Source: CAD feature listing. Evaluate the final solid. Frame: model axes, mm. Face numbers are marked on the shaded views. A direction names the side the tool comes from. Round coordinates to 2 decimals unless told otherwise and drop trailing zeros. Order: outer loops, then holes, each group sorted by start corner. A loop starts at its lowest first (then second) coordinate and runs counter-clockwise, first axis right, second up. Notation, with made-up numbers: (60, -10) -> (89, -10) arc R18 cw to (89, 11) -> close; hole circle Ø5 at (79, 78.25). An arc over 180 degrees is marked (long way). One line per item, written item: value. Start each with the question number.
1) Section C-C (y = 7.5). Return the cut outline in (x, z), and give its area (3 significant figures).
2) Ray query, L1, parallel to Y at x = 2, z = 6.5; L2, parallel to Y at x = -1.75, z = 4.25; L3, parallel to Z at x = -5, y = -6. Return the intervals inside material, ascending.
3) Section B-B (z = 5.25). Return the cut outline in (x, y).
4) Reachability of the marked faces 1, 2, 3, 4 and 5 from +Z, -Z, +X, -X, +Y, -Y: full face, straight path, thin tool, end or side. Return the list, or none.
5) Section A-A (x = 4). Return the cut outline in (y, z).
6) Pin query (flat end, axial travel): P1, Ø2.5, axis at y = -9.5, z = 4.5, coming from the +X side; P2, Ø8, axis at x = -1.5, z = 13.5, coming from the -Y side; P3, Ø5.5, axis at x = -3, z = 5, coming from the +Y side; P4, Ø1.1, axis at y = 9.5, z = 6.5, coming from the -X side. Return the tip coordinate at first contact, or that it passes through.
7) Section D-D (x = 1.5). Return the cut outline in (y, z).
8) Mould query, pull axis Y, two halves, no side actions, for the marked faces 6, 7, 8 and 9. Classes: pulls with the +Y half, pulls with the -Y half, needs draft (parallel to the pull), parting line crosses it, or undercut.
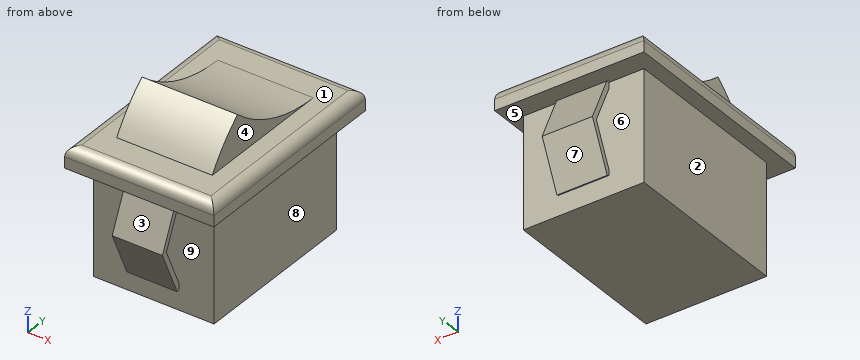
```python
from build123d import *

# Parameters (mm, degrees)
ESQUISSE1_W        = 12
ESQUISSE1_H        = 17
BOSS_EXTRU_1_DEPTH = 11
ESQUISSE2_W        = 14.823529412
ESQUISSE2_H        = 21
BOSS_EXTRU_2_DEPTH = 2.1
BOSS_EXTRU_3_DEPTH = 4.75
EXTRU_MINCE1_DEPTH = 2.5
CONG_1_R           = 1


with BuildPart() as part:
    # Esquisse1 → Boss.-Extru.1 (new body)
    with BuildSketch(Plane.XY):
        Rectangle(ESQUISSE1_W, ESQUISSE1_H)
    extrude(amount=BOSS_EXTRU_1_DEPTH)

    # Esquisse2 → Boss.-Extru.2 (add)
    with BuildSketch(Plane.XY.offset(11)):
        Rectangle(ESQUISSE2_W, ESQUISSE2_H)
    extrude(amount=BOSS_EXTRU_2_DEPTH)

    # Esquisse3 → Boss.-Extru.3 (add, symmetric)
    with BuildSketch(Plane(origin=(0, 0, 0), x_dir=(0, 0, -1), z_dir=(1, 0, 0))):
        with BuildLine():
            Line((-13.1, -7), (-13.1, 7))
            ThreePointArc((-13.1, 7), (-14.133865433, 1.381948736), (-17.1, -3.5))
            ThreePointArc((-17.1, -3.5), (-15.248408263, -5.419609444), (-13.1, -7))
        make_face()
    extrude(amount=BOSS_EXTRU_3_DEPTH, both=True)

    # Esquisse4 → Extru.-Mince1 (add, symmetric)
    with BuildSketch(Plane(origin=(0, 0, 0), x_dir=(0, 0, -1), z_dir=(1, 0, 0))):
        Polygon((-11.101534617, -8.728452887), (-6.5, -10.773579383), (-1.898465383, -8.728452887), (-2.101534617, -8.271547113), (-6.5, -10.226420617), (-10.898465383, -8.271547113), align=None)
        Polygon((-10.898465383, 8.271547113), (-6.5, 10.226420617), (-2.101534617, 8.271547113), (-1.898465383, 8.728452887), (-6.5, 10.773579383), (-11.101534617, 8.728452887), align=None)
    extrude(amount=EXTRU_MINCE1_DEPTH, both=True)

    # Congé1
    cong_1_edges = [part.edges().sort_by_distance(p)[0] for p in [
        (7.411764706, 0, 13.1),
        (0, 10.5, 13.1),
        (-7.411764706, 0, 13.1),
        (0, -10.5, 13.1),
    ]]
    fillet(cong_1_edges, radius=CONG_1_R)


solid = part.part
```
Findings:
1. outline: (-7.41, 11) -> (-6, 11) -> (-6, 0) -> (6, 0) -> (6, 11) -> (7.41, 11) -> (7.41, 12.1) arc R1 ccw to (6.41, 13.1) -> (-6.41, 13.1) arc R1 ccw to (-7.41, 12.1) -> close
1. area: 163 mm2
2. L1: -10.77 to -10.23, -8.5 to 8.5, 10.23 to 10.77
2. L2: -9.77 to -9.23, -8.5 to 8.5, 9.23 to 9.77
2. L3: 0 to 13.1
3. outline: (-6, -8.5) -> (6, -8.5) -> (6, 8.5) -> (-6, 8.5) -> close; (-2.5, -10.22) -> (2.5, -10.22) -> (2.5, -9.67) -> (-2.5, -9.67) -> close; (-2.5, 9.67) -> (2.5, 9.67) -> (2.5, 10.22) -> (-2.5, 10.22) -> close
4. face 1: +Z
4. face 2: -Z, -X, +Y, -Y
4. face 3: +X, -X, -Y
4. face 4: +Z, +X, +Y, -Y
4. face 5: none
5. outline: (-10.5, 11) -> (-8.5, 11) -> (-8.5, 0) -> (8.5, 0) -> (8.5, 11) -> (10.5, 11) -> (10.5, 12.1) arc R1 ccw to (9.5, 13.1) -> (7, 13.1) arc R15.78 cw to (-3.5, 17.1) arc R15.78 ccw to (-7, 13.1) -> (-9.5, 13.1) arc R1 ccw to (-10.5, 12.1) -> close
6. P1: x = 6
6. P2: y = -10.5
6. P3: y = 10.77
6. P4: through
7. outline: (-10.77, 6.5) -> (-8.73, 1.9) -> (-8.5, 2) -> (-8.5, 0) -> (8.5, 0) -> (8.5, 2) -> (8.73, 1.9) -> (10.77, 6.5) -> (8.77, 11) -> (10.5, 11) -> (10.5, 12.1) arc R1 ccw to (9.5, 13.1) -> (7, 13.1) arc R15.78 cw to (-3.5, 17.1) arc R15.78 ccw to (-7, 13.1) -> (-9.5, 13.1) arc R1 ccw to (-10.5, 12.1) -> (-10.5, 11) -> (-8.77, 11) -> close; hole (-10.23, 6.5) -> (-8.5, 2.62) -> (-8.5, 10.38) -> close; hole (8.5, 2.62) -> (10.23, 6.5) -> (8.5, 10.38) -> close
8. face 6: undercut
8. face 7: pulls with the +Y half
8. face 8: needs draft
8. face 9: undercut
